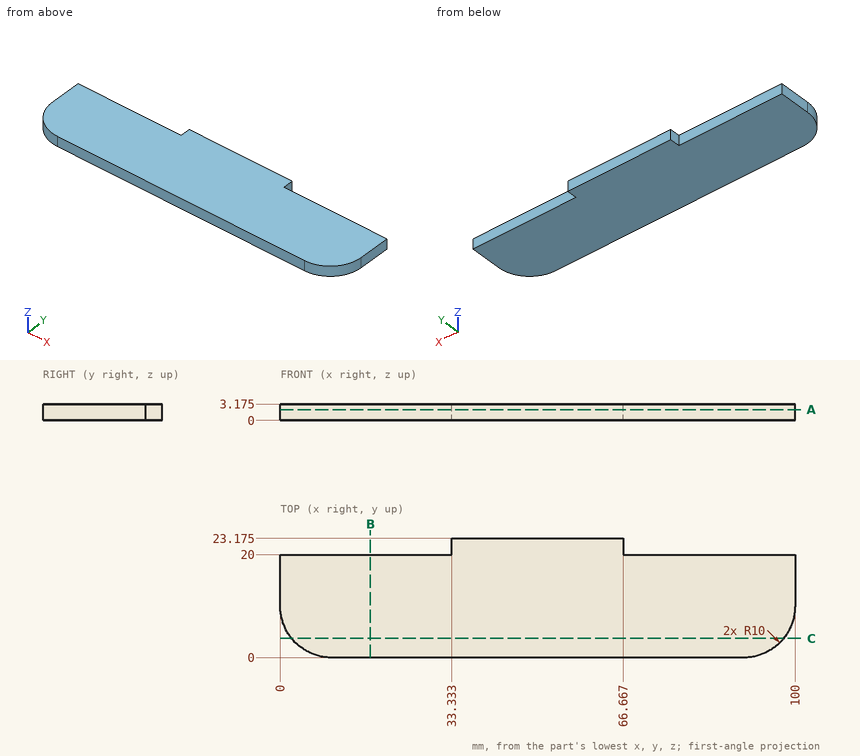
Print and shaded views of the part. All mm, measured from the part's lowest x, y and z. Coordinates: 2 decimals unless noted, no trailing zeros. Write each loop counter-clockwise with the first axis right and the second up, starting at its lowest first coordinate (ties: lowest second). Pieces come first, ordered by that corner, then holes.
(1) Cut at B-B, the plane x = 17.5. List the corners of the cut face in (y, z) (1 decimal).
(2) Flat gauge pins, fed straight in: pin 1 (1 mm diameter, centred on x = 13.5, z = 2, fed in from +Y); pin 2 (1 mm diameter, centred on y = 22, z = 2, fed in from -X); pin 3 (1 mm diameter, centred on y = 22, z = 2, fed in from +X). Where does each tip first touch, or does it go through?
(3) Drill centre lines: probe 1 along Y at (x, z) = (32.5, 1.45); probe 2 along X at (y, z) = (20.25, 0.5); probe 3 along X at (y, z) = (4.75, 2.5). Where is each one in solid material? Low to high.
(4) Cut at C-C, the plane y = 3.75. List the corners of the cut face in (x, z) (1 decimal).
(5) Cut at A-A, the plane z = 2.1. List the corners of the cut face in (x, y) (1 decimal), and give its area (3 significant figures).
Geometry says:
1. outline: (0, 0) - (20, 0) - (20, 3.2) - (0, 3.2) - close
2. pin 1: stops at y = 20
2. pin 2: stops at x = 33.33
2. pin 3: stops at x = 66.67
3. probe 1: y = 0 to 20
3. probe 2: x = 33.33 to 66.67
3. probe 3: x = 1.49 to 98.51
4. outline: (2.2, 0) - (97.8, 0) - (97.8, 3.2) - (2.2, 3.2) - close
5. outline: (0, 10) arc R10 ccw to (10, 0) - (90, 0) arc R10 ccw to (100, 10) - (100, 20) - (66.7, 20) - (66.7, 23.2) - (33.3, 23.2) - (33.3, 20) - (0, 20) - close
5. area: 2,060 mm2
